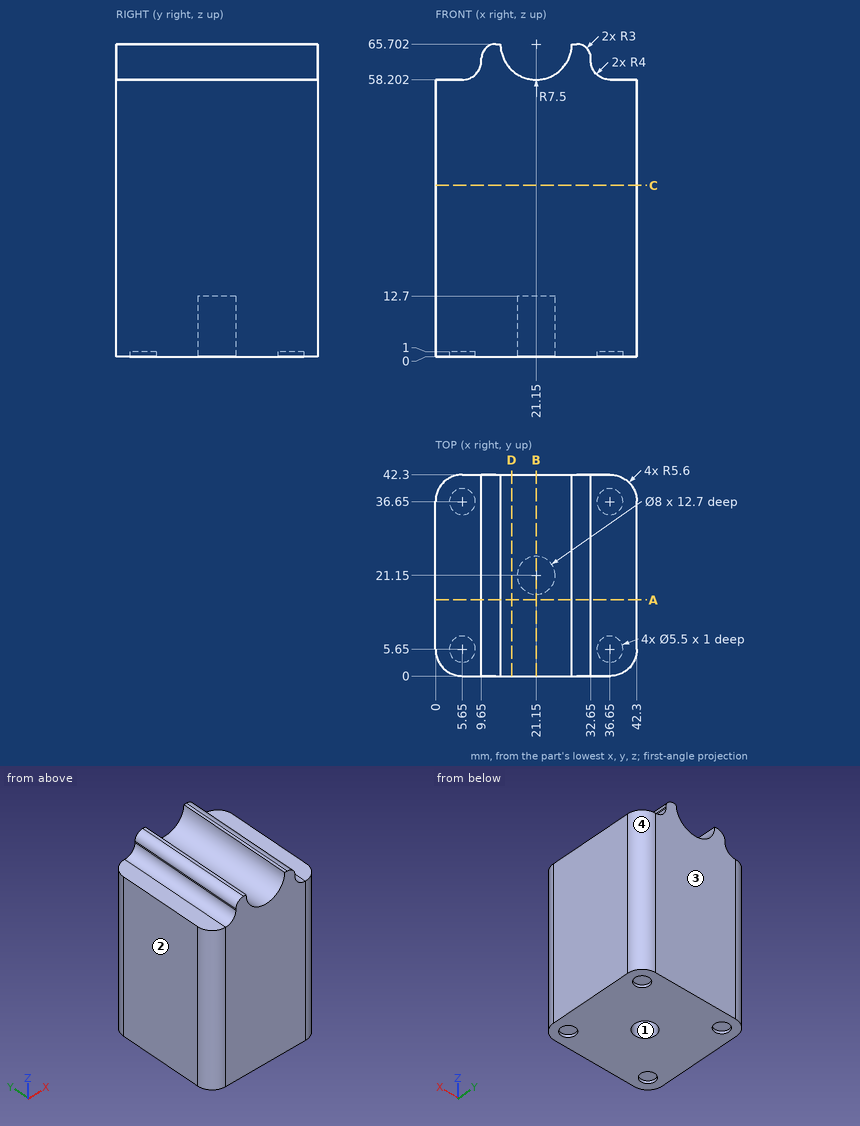
Check sheet for the drawn part. Datum: minimum x, y, z corner. Units: mm. Round coordinates to 2 decimals unless told otherwise and drop trailing zeros. Loops run counter-clockwise (first coordinate to the right, second up) from the corner with the lowest first, then second, coordinate; pieces in that order, holes last.
Item 1: Cross-section at A-A on y = 16. Record the boundary of the cut face in (x, z).
Item 2: Thickness scan on line 1 (Y direction, x = 5.65, z = 0.55); line 2 (Y direction, x = 21, z = 7); line 3 (Z direction, x = 21, y = 40). Record the ranges inside material, lowest first.
Item 3: Cross-section at B-B on x = 21.15. Record the boundary of the cut face in (y, z), then the cut area to 3 significant figures.
Item 4: Mould release check, pull along X, two halves, no side actions. Record for the marked faces 1, 2, 3 and 4: pulls with the +X half, pulls with the -X half, needs draft (parallel to the pull), parting line crosses it, or undercut.
Item 5: Gauge pin test, flat ends, axial feed: pin 1 (0.6 mm diameter, centred on y = 25, z = 62.5, fed in from -X); pin 2 (1 mm diameter, centred on x = 10, y = 36, fed in from +Z) (1 decimal); pin 3 (5 mm diameter, centred on x = 12, z = 39, fed in from -Y); pin 4 (6 mm diameter, centred on x = 4, y = 24, fed in from +Z). Record the tip position at first contact, or that the pin passes through.
Item 6: Cross-section at C-C on z = 36. Record the boundary of the cut face in (x, y), then the cut area to 3 significant figures.
Item 7: Cross-section at D-D on x = 16. Record the boundary of the cut face in (y, z).
Answer sheet:
1. outline: (0, 0) - (42.3, 0) - (42.3, 58.2) - (36.65, 58.2) arc R4 cw to (32.65, 62.2) - (32.65, 62.7) arc R3 ccw to (29.65, 65.7) - (28.65, 65.7) arc R7.5 cw to (13.65, 65.7) - (12.65, 65.7) arc R3 ccw to (9.65, 62.7) - (9.65, 62.2) arc R4 cw to (5.65, 58.2) - (0, 58.2) - close
2. line 1: y = 0 to 2.9, 8.4 to 33.9, 39.4 to 42.3
2. line 2: y = 0 to 17.15, 25.15 to 42.3
2. line 3: z = 0 to 58.2
3. outline: (0, 0) - (17.15, 0) - (17.15, 12.7) - (25.15, 12.7) - (25.15, 0) - (42.3, 0) - (42.3, 58.2) - (0, 58.2) - close
3. area: 2,360 mm2
4. face 1: undercut
4. face 2: pulls with the -X half
4. face 3: needs draft
4. face 4: pulls with the +X half
5. pin 1: stops at x = 9.65
5. pin 2: stops at z = 64.8
5. pin 3: stops at y = 0
5. pin 4: stops at z = 58.44
6. outline: (0, 5.6) arc R5.6 ccw to (5.6, 0) - (36.7, 0) arc R5.6 ccw to (42.3, 5.6) - (42.3, 36.7) arc R5.6 ccw to (36.7, 42.3) - (5.6, 42.3) arc R5.6 ccw to (0, 36.7) - close
6. area: 1,760 mm2
7. outline: (0, 0) - (42.3, 0) - (42.3, 60.25) - (0, 60.25) - close
